Model file for the job. Use its own axes, mm. Face numbers are marked on the shaded views. A direction names the side the tool comes from. Give positions to 0.01 mm unless a question says otherwise; leave off trailing zeros. Order: outer loops, then holes, each group sorted by start corner. A loop starts at its lowest first (then second) coordinate and runs counter-clockwise, first axis right, second up. Notation, with made-up numbers: (31, -22.5) - (56, -22.5) arc R18 ccw to (56, -9.5) - close; hole circle Ø11 at (18.5, -8). An arc over 180 degrees is marked (long way). Return JSON: item names as keys, results as strings. Group by question number.
from build123d import *

# Parameters (mm, degrees)
PAD_DEPTH       = 18
POCKET_DEPTH    = 16
POCKET001_DEPTH = 5


with BuildPart() as part:
    # Sketch → Pad (new body)
    with BuildSketch(Plane.XY):
        with BuildLine():
            Line((-13.5, -16.5), (13.5, -16.5))
            ThreePointArc((13.5, -16.5), (18.449747, -14.449747), (20.5, -9.5))
            Line((20.5, -9.5), (20.5, 9.5))
            ThreePointArc((20.5, 9.5), (18.449747, 14.449747), (13.5, 16.5))
            Line((13.5, 16.5), (-13.5, 16.5))
            ThreePointArc((-13.5, 16.5), (-18.449747, 14.449747), (-20.5, 9.5))
            Line((-20.5, 9.5), (-20.5, -9.5))
            ThreePointArc((-20.5, -9.5), (-18.449747, -14.449747), (-13.5, -16.5))
        make_face()
    extrude(amount=PAD_DEPTH)

    # Sketch001 (on Face10 of Pad) → Pocket (cut)
    with BuildSketch(Plane.XY.offset(18)):
        with BuildLine():
            Line((-18.5, 11), (-18.5, -11))
            ThreePointArc((-18.5, -11), (-17.328427, -13.828427), (-14.5, -15))
            Line((-14.5, -15), (14.5, -15))
            ThreePointArc((14.5, -15), (17.328427, -13.828427), (18.5, -11))
            Line((18.5, -11), (18.5, 11))
            ThreePointArc((18.5, 11), (17.328427, 13.828427), (14.5, 15))
            Line((14.5, 15), (-14.5, 15))
            ThreePointArc((-14.5, 15), (-17.328427, 13.828427), (-18.5, 11))
        make_face()
    extrude(amount=-POCKET_DEPTH, mode=Mode.SUBTRACT)

    # Sketch002 (on Face1 of Pocket) → Pocket001 (cut)
    with BuildSketch(Plane.XZ.offset(16.5)):
        with BuildLine():
            Line((-6, 24), (-6, 4))
            ThreePointArc((-6, 4), (-5.414214, 2.585786), (-4, 2))
            Line((-4, 2), (2, 2))
            ThreePointArc((2, 2), (3.414214, 2.585786), (4, 4))
            Line((4, 4), (4, 24))
            ThreePointArc((4, 24), (3.414214, 25.414214), (2, 26))
            Line((2, 26), (-4, 26))
            ThreePointArc((-4, 26), (-5.414214, 25.414214), (-6, 24))
        make_face()
    extrude(amount=-POCKET001_DEPTH, mode=Mode.SUBTRACT)


solid = part.part
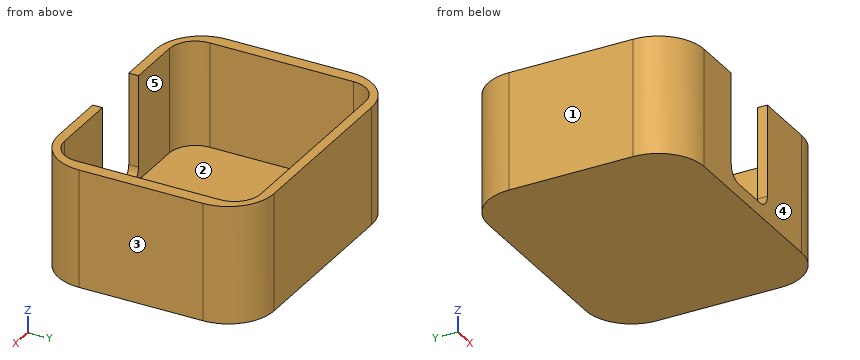
(1) Drill centre lines: L1, parallel to Y at x = -12, z = 11.25; L2, parallel to X at y = -7, z = 17.25; L3, parallel to Z at x = -9.5, y = -13.5. Where is each one in solid material? Low to high.
(2) Slice it at B-B (z = 15.5). Give the cut face in (x, y), and give its area (3 significant figures).
(3) 3-axis set-ups, long thin cutter, end or side, ignore diameter. For the marked faces 1 and 2: which of +Z, -Z, +X, -X, +Y, -Y reach the whole face in a straight line?
(4) Slice it at D-D (z = 2.75). Give the cut face in (x, y), and give its area (3 significant figures).
(5) Drop flat-ended pins along their axis: pin 1 Ø1 at (x, z) = (-15, 2.5) entering from +Y; pin 2 Ø2 at (x, y) = (16, -9.5) entering from +Z; pin 3 Ø1.2 at (y, z) = (-16, 9) entering from -X; pin 4 Ø10 at (x, y) = (-3.5, 11) entering from +Z. Give the stop position or say it passes through.
(6) Slice it at C-C (y = 3.5). Give the cut face in (x, z), and give its area (3 significant figures).
(7) Slice it at A-A (x = 6). Give the cut face in (y, z), and give its area (3 significant figures).
(8) Pull direction X, two halves, no side cores. Call the marked faces 3, 4 and 5: released by +X, released by -X, zero draft, split by the parting line, or undercut.
Result set:
{
 "1": {"L1": "y = -16.5 to -15, 15 to 16.5", "L2": "x = -20.5 to -18.5, 18.5 to 20.5", "L3": "z = 0 to 2"},
 "2": {"outline": "(-20.5, -9.5) arc R7 ccw to (-13.5, -16.5) - (-6, -16.5) - (-6, -15) - (-14.5, -15) arc R4 cw to (-18.5, -11) - (-18.5, 11) arc R4 cw to (-14.5, 15) - (14.5, 15) arc R4 cw to (18.5, 11) - (18.5, -11) arc R4 cw to (14.5, -15) - (4, -15) - (4, -16.5) - (13.5, -16.5) arc R7 ccw to (20.5, -9.5) - (20.5, 9.5) arc R7 ccw to (13.5, 16.5) - (-13.5, 16.5) arc R7 ccw to (-20.5, 9.5) - close", "area": "200 mm²"},
 "3": {"face 1": "+Z, -Z, -X, +Y, -Y", "face 2": "+Z"},
 "4": {"outline": "(-20.5, -9.5) arc R7 ccw to (-13.5, -16.5) - (-5.56, -16.5) - (-5.56, -15) - (-14.5, -15) arc R4 cw to (-18.5, -11) - (-18.5, 11) arc R4 cw to (-14.5, 15) - (14.5, 15) arc R4 cw to (18.5, 11) - (18.5, -11) arc R4 cw to (14.5, -15) - (3.56, -15) - (3.56, -16.5) - (13.5, -16.5) arc R7 ccw to (20.5, -9.5) - (20.5, 9.5) arc R7 ccw to (13.5, 16.5) - (-13.5, 16.5) arc R7 ccw to (-20.5, 9.5) - close", "area": "201 mm²"},
 "5": {"pin 1": "stops at y = 16.43", "pin 2": "stops at z = 2", "pin 3": "stops at x = -17.27", "pin 4": "stops at z = 18"},
 "6": {"outline": "(-20.5, 0) - (20.5, 0) - (20.5, 18) - (18.5, 18) - (18.5, 2) - (-18.5, 2) - (-18.5, 18) - (-20.5, 18) - close", "area": "146 mm²"},
 "7": {"outline": "(-16.5, 0) - (16.5, 0) - (16.5, 18) - (15, 18) - (15, 2) - (-15, 2) - (-15, 18) - (-16.5, 18) - close", "area": "114 mm²"},
 "8": {"face 3": "released by +X", "face 4": "zero draft", "face 5": "undercut"}
}
